Here's how the part is built. I have some questions about the finished solid (model axes, mm). Give positions to 0.01 mm unless a question says otherwise; leave off trailing zeros. Write each loop counter-clockwise with the first axis right and the second up, starting at its lowest first coordinate (ties: lowest second). Pieces come first, ordered by that corner, then holes. Notation, with made-up numbers: (45, 44) -> (51, 44) arc R27 ccw to (51, 62) -> close; hole circle Ø9 at (-12.5, 14). An arc over 180 degrees is marked (long way). Use one line per item in the form item = value.
```python
from build123d import *

# Parameters (mm, degrees)
SKETCH_1_R      = 13.5
SKETCH_1_R_2    = 4
SKETCH_1_R_3    = 1.5
EXTRUDE_1_DEPTH = 1.5
SKETCH_1_4_R    = 6
SKETCH_1_4_R_2  = 4
EXTRUDE_2_DEPTH = 12


with BuildPart() as part:
    # Sketch 1 → Extrude 1 (new body)
    with BuildSketch(Plane.XY):
        Circle(SKETCH_1_R)
        Circle(SKETCH_1_R_2, mode=Mode.SUBTRACT)
        with Locations((8.227241336, -4.75)):
            Circle(SKETCH_1_R_3, mode=Mode.SUBTRACT)
        with Locations((-8.227241336, -4.75)):
            Circle(SKETCH_1_R_3, mode=Mode.SUBTRACT)
        with Locations((0, 9.5)):
            Circle(SKETCH_1_R_3, mode=Mode.SUBTRACT)
    extrude(amount=EXTRUDE_1_DEPTH)

    # Sketch 1_4 → Extrude 2 (add)
    with BuildSketch(Plane.XY):
        Circle(SKETCH_1_4_R)
        Circle(SKETCH_1_4_R_2, mode=Mode.SUBTRACT)
    extrude(amount=EXTRUDE_2_DEPTH)


solid = part.part
```
Q1. I want a section at C-C, the plane y = -4.75. Write out the boundary of the cut face in (x, z).
Result set:
outline = (-12.64, 0) -> (-9.73, 0) -> (-9.73, 1.5) -> (-12.64, 1.5) -> close; (-6.73, 0) -> (6.73, 0) -> (6.73, 1.5) -> (3.67, 1.5) -> (3.67, 12) -> (-3.67, 12) -> (-3.67, 1.5) -> (-6.73, 1.5) -> close; (9.73, 0) -> (12.64, 0) -> (12.64, 1.5) -> (9.73, 1.5) -> close
Q2. Will these pins go through, and if not, where does the flat tip stop? pin 1 Ø7 at (x, y) = (0, 0) entering from +Z; pin 2 Ø4 at (x, y) = (-10, 10) entering from +Z; pin 3 Ø4 at (y, z) = (7, 6) entering from -X.
Result set:
pin_1 = through
pin_2 = 1.5
pin_3 = -3.32
Q3. I want a section at A-A, the plane x = 0. Write out the boundary of the cut face in (y, z), and give its area (3 significant figures).
Result set:
outline = (-13.5, 0) -> (-4, 0) -> (-4, 12) -> (-6, 12) -> (-6, 1.5) -> (-13.5, 1.5) -> close; (4, 0) -> (8, 0) -> (8, 1.5) -> (6, 1.5) -> (6, 12) -> (4, 12) -> close; (11, 0) -> (13.5, 0) -> (13.5, 1.5) -> (11, 1.5) -> close
area = 66.0 mm2
Q4. I want a section at B-B, the plane y = 0. Write out the boundary of the cut face in (x, z), and give its area (3 significant figures).
Result set:
outline = (-13.5, 0) -> (-4, 0) -> (-4, 12) -> (-6, 12) -> (-6, 1.5) -> (-13.5, 1.5) -> close; (4, 0) -> (13.5, 0) -> (13.5, 1.5) -> (6, 1.5) -> (6, 12) -> (4, 12) -> close
area = 70.5 mm2
Q5. If we mould it in two halves opening along Y, with no side actions, what happens to faces 1 (the face through (-6, 0, 7)), 2 (the face through (-9.726, -4.684, 0.74)), 3 (the face through (6, -3, 1.5))? For each: +Y half, -Y half, draft (parallel to the pull), parting line (faces both ways), or undercut.
Result set:
face_1 = parting line
face_2 = undercut
face_3 = draft
Q6. I want a section at D-D, the plane x = -8.25. Write out the boundary of the cut face in (y, z), and give its area (3 significant figures).
Result set:
outline = (-10.69, 0) -> (-6.25, 0) -> (-6.25, 1.5) -> (-10.69, 1.5) -> close; (-3.25, 0) -> (10.69, 0) -> (10.69, 1.5) -> (-3.25, 1.5) -> close
area = 27.6 mm2
Q7. If I drill on line 1 along Y through (x, z) = (0, 0.8); line 2 along Y through (x, z) = (-1, 6); line 3 along Z through (x, y) = (7.5, 7.5), over which ranges is the centre line in solid material (lowest first)? Write a range as from..to.
Result set:
line_1 = -13.5..-4, 4..8, 11..13.5
line_2 = -5.92..-3.87, 3.87..5.92
line_3 = 0..1.5
